Can you work these out from the model? Positions are in its coordinate system, mm. Face numbers are marked on the shaded views. A direction names the side the tool comes from. Coordinates: 2 decimals unless noted, no trailing zeros. Order: outer loops, then holes, each group sorted by start corner. A loop starts at its lowest first (then second) coordinate and runs counter-clockwise, first axis right, second up. Notation, with made-up numbers: (-6.5, -20) -> (14.5, -20) arc R21 ccw to (14.5, -10) -> close; hole circle Ø1 at (88.25, -16). An arc over 180 degrees is marked (long way). Use a Markdown table: item, result. Add a question column.
1. If I drill on line 1 along X through (y, z) = (88.5, 14.75); line 2 along X through (y, z) = (86, 2.75); line 3 along X through (y, z) = (89.5, 4), over which ranges is the centre line in solid material (lowest first)? Write a range as from..to.
2. Suppose I cut it at B-B, the plane z = 17.5. State how many separate pieces and enclosed holes the cut face has, then the cut area to 3 significant figures.
3. For the marked faces 4, 5 and 6, which set-ups out of +Z, -Z, +X, -X, +Y, -Y let a thin tool reach every point of the face, with its end or its side?
4. For pin 1 Ø6 at (y, z) = (92, 15.5) entering from -X; pin 2 Ø3.5 at (x, z) = (12.5, 7) entering from +Y; pin 3 Ø1.5 at (y, z) = (8, 18.5) entering from +X, each with a flat end and sliding along its axis, tell me the tip position at first contact or that it passes through.
5. Suppose I cut it at A-A, the plane y = 115. List the corners of the cut face in (x, z) for me.
6. We'd pull the mould along X, two halves only. Please class the marked faces 1, 2 and 3: pulls with the +X half, pulls with the -X half, needs draft (parallel to the pull), parting line crosses it, or undercut.
```python
from build123d import *

# Parameters (mm, degrees)
BOSS_EXTRUDE1_DEPTH = 25
SKETCH3_W           = 36
SKETCH3_H           = 10
CUT_EXTRUDE1_DEPTH  = 134.88427839
CUT_EXTRUDE2_DEPTH  = 134.88427839
CUT_EXTRUDE3_DEPTH  = 134.88427839
CUT_EXTRUDE4_DEPTH  = 134.88427839
BOSS_EXTRUDE2_DEPTH = 25
BOSS_EXTRUDE3_DEPTH = 25
LPATTERN1_COUNT     = 30
LPATTERN1_PITCH     = 3
CUT_EXTRUDE5_DEPTH  = 138.359842306
CUT_EXTRUDE6_DEPTH  = 138.359842306
CUT_EXTRUDE7_DEPTH  = 138.359842306
CUT_EXTRUDE8_DEPTH  = 138.359842306
CUT_EXTRUDE9_DEPTH  = 138.359842306
FILLET1_R           = 1


with BuildPart() as part:
    # Sketch2 → Boss-Extrude1 (new body)
    with BuildSketch(Plane.XY):
        with BuildLine():
            Line((-15, 0), (15, 0))
            Line((15, 0), (15, 5))
            Line((15, 5), (8, 5))
            Line((8, 5), (8, 10))
            Line((8, 10), (20, 10))
            Line((20, 10), (20, 130))
            ThreePointArc((20, 130), (-9.083269132, 106.055512755), (-20, 70))
            Line((-20, 70), (-20, 10))
            Line((-20, 10), (-8, 10))
            Line((-8, 10), (-8, 5))
            Line((-8, 5), (-15, 5))
            Line((-15, 5), (-15, 0))
        make_face()
    extrude(amount=BOSS_EXTRUDE1_DEPTH)

    # Sketch3 → Cut-Extrude1 (cut, through all)
    with BuildSketch(Plane.XY.offset(25)):
        with Locations((0, 17)):
            Rectangle(SKETCH3_W, SKETCH3_H)
    extrude(amount=-CUT_EXTRUDE1_DEPTH, mode=Mode.SUBTRACT)

    # Sketch4 → Cut-Extrude2 (cut, through all)
    with BuildSketch(Plane.XY.offset(25)):
        Polygon((-18, 24), (18, 24), (18, 34), (-18, 40.347771306), align=None)
    extrude(amount=-CUT_EXTRUDE2_DEPTH, mode=Mode.SUBTRACT)

    # Sketch5 → Cut-Extrude3 (cut, through all)
    with BuildSketch(Plane.XY.offset(25)):
        Polygon((-18, 42.378624529), (18, 36.030853224), (18, 46.030853224), (-18, 59.133781657), align=None)
    extrude(amount=-CUT_EXTRUDE3_DEPTH, mode=Mode.SUBTRACT)

    # Sketch6 → Cut-Extrude4 (cut, through all)
    with BuildSketch(Plane.XY.offset(25)):
        with BuildLine():
            Line((-18, 61.262137202), (18, 48.159208769))
            Line((18, 48.159208769), (18, 58.159208769))
            Line((18, 58.159208769), (-17.409830527, 78.603083956))
            ThreePointArc((-17.409830527, 78.603083956), (-17.852284458, 74.311651469), (-18, 70))
            Line((-18, 70), (-18, 61.262137202))
        make_face()
    extrude(amount=-CUT_EXTRUDE4_DEPTH, mode=Mode.SUBTRACT)

    # Sketch13 → Boss-Extrude2 (add)
    with BuildSketch(Plane.XY.offset(25)):
        with BuildLine():
            Line((28.543587015, 132.015112463), (28.543587015, 130.015112463))
            ThreePointArc((28.543587015, 130.015112463), (22.183163486, 116.610368534), (20, 101.934676234))
            Line((20, 101.934676234), (20, 130))
            ThreePointArc((20, 130), (24.189413282, 131.356828362), (28.543587015, 132.015112463))
        make_face()
    extrude(amount=-BOSS_EXTRUDE2_DEPTH)

    # Sketch15 → Boss-Extrude3 (add)
    with BuildSketch(Plane.XY.offset(25)):
        Polygon((20, 101.934676234), (22.598076211, 100.434676234), (20, 98.934676234), align=None)
    boss_extrude3 = extrude(amount=-BOSS_EXTRUDE3_DEPTH)

    # LPattern1: Boss-Extrude3 ×30
    with Locations(*[(0, -i * LPATTERN1_PITCH, 0) for i in range(1, LPATTERN1_COUNT)]):
        add(boss_extrude3)

    # Sketch17 → Cut-Extrude5 (cut, through all)
    with BuildSketch(Plane.XY.offset(25)):
        with BuildLine():
            Line((-17.080813578, 80.722527008), (18, 60.468609845))
            Line((18, 60.468609845), (18, 70.468609845))
            Line((18, 70.468609845), (-12.396357526, 95.974182235))
            ThreePointArc((-12.396357526, 95.974182235), (-15.223349712, 88.497247077), (-17.080813578, 80.722527008))
        make_face()
    extrude(amount=-CUT_EXTRUDE5_DEPTH, mode=Mode.SUBTRACT)

    # Sketch18 → Cut-Extrude6 (cut, through all)
    with BuildSketch(Plane.XY.offset(25)):
        with BuildLine():
            Line((-11.513032555, 97.843799156), (18, 73.079424424))
            Line((18, 73.079424424), (18, 83.079424424))
            Line((18, 83.079424424), (-4.123287406, 109.44493167))
            ThreePointArc((-4.123287406, 109.44493167), (-8.135718614, 103.846645438), (-11.513032555, 97.843799156))
        make_face()
    extrude(amount=-CUT_EXTRUDE6_DEPTH, mode=Mode.SUBTRACT)

    # Sketch19 → Cut-Extrude7 (cut, through all)
    with BuildSketch(Plane.XY.offset(25)):
        with BuildLine():
            Line((-2.825102167, 111.009262402), (18, 86.190872078))
            Line((18, 86.190872078), (18, 96.190872078))
            Line((18, 96.190872078), (5.013768012, 118.68368568))
            ThreePointArc((5.013768012, 118.68368568), (0.926972027, 115.017421131), (-2.825102167, 111.009262402))
        make_face()
    extrude(amount=-CUT_EXTRUDE7_DEPTH, mode=Mode.SUBTRACT)

    # Sketch21 → Cut-Extrude8 (cut, through all)
    with BuildSketch(Plane.XY.offset(25)):
        with BuildLine():
            Line((6.596754137, 119.941873284), (18, 100.190872078))
            Line((18, 100.190872078), (18, 110.190872078))
            Line((18, 110.190872078), (12.898276405, 124.207742456))
            ThreePointArc((12.898276405, 124.207742456), (9.683048128, 122.170038436), (6.596754137, 119.941873284))
        make_face()
    extrude(amount=-CUT_EXTRUDE8_DEPTH, mode=Mode.SUBTRACT)

    # Sketch22 → Cut-Extrude9 (cut, through all)
    with BuildSketch(Plane.XY.offset(25)):
        with BuildLine():
            Line((14.660598632, 125.213410732), (18, 116.038480878))
            Line((18, 116.038480878), (18, 126.920997883))
            ThreePointArc((18, 126.920997883), (16.317589, 126.092060929), (14.660598632, 125.213410732))
        make_face()
    extrude(amount=-CUT_EXTRUDE9_DEPTH, mode=Mode.SUBTRACT)

    # Fillet1
    fillet1_edges = [part.edges().sort_by_distance(p)[0] for p in [
        (18, 70.468609845, 12.5),
        (18, 60.468609845, 12.5),
        (-17.080813578, 80.722527008, 12.5),
        (-12.396357526, 95.974182235, 12.5),
        (-11.513032555, 97.843799156, 12.5),
        (-4.123287406, 109.44493167, 12.5),
        (18, 83.079424424, 12.5),
        (18, 73.079424424, 12.5),
        (18, 96.190872078, 12.5),
        (18, 86.190872078, 12.5),
        (-2.825102167, 111.009262402, 12.5),
        (5.013768012, 118.68368568, 12.5),
        (6.596754137, 119.941873284, 12.5),
        (12.898276405, 124.207742456, 12.5),
        (18, 110.190872078, 12.5),
        (18, 100.190872078, 12.5),
        (14.660598632, 125.213410732, 12.5),
        (18, 126.920997883, 12.5),
        (18, 116.038480878, 12.5),
        (-18, 12, 12.5),
        (-18, 22, 12.5),
        (18, 22, 12.5),
        (18, 12, 12.5),
        (-18, 24, 12.5),
        (-18, 40.347771306, 12.5),
        (18, 34, 12.5),
        (18, 24, 12.5),
        (-18, 42.378624529, 12.5),
        (-18, 59.133781657, 12.5),
        (18, 46.030853224, 12.5),
        (18, 36.030853224, 12.5),
        (-18, 61.262137202, 12.5),
        (-17.409830527, 78.603083956, 12.5),
        (18, 58.159208769, 12.5),
        (18, 48.159208769, 12.5),
    ]]
    fillet(fillet1_edges, radius=FILLET1_R)


solid = part.part
```
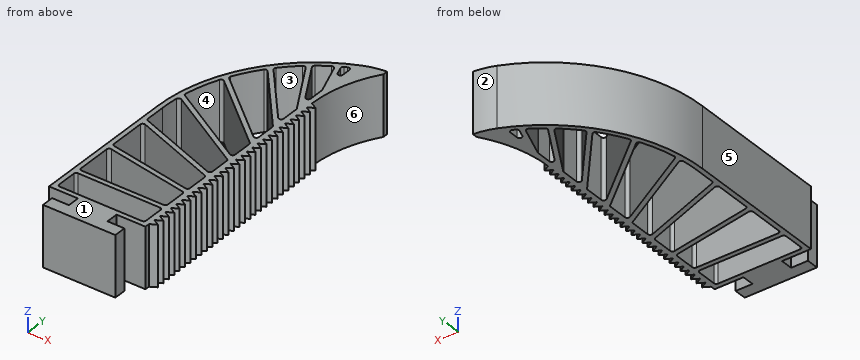
Worked out:
| question | item | result |
|---|---|---|
| 1 | line 1 | x = -17.31..-15.22, -3.49..-0.38, 13.45..16.06, 17.9..22.48 |
| 1 | line 2 | x = -18..-15.93, -0.51..2.6, 15.55..21.62 |
| 1 | line 3 | x = -17.01..-14.91, -4.68..-1.57, 12.61..15.22, 18..20.75 |
| 2 | separate pieces | 1 |
| 2 | enclosed holes | 9 |
| 2 | area | 1,550 mm² |
| 3 | face 4 | +Z, -Z |
| 3 | face 5 | +Z, -Z, -X, +Y, -Y |
| 3 | face 6 | +Z, -Z, +X |
| 4 | pin 1 | stops at x = -17.16 |
| 4 | pin 2 | stops at y = 127.27 |
| 4 | pin 3 | stops at x = 8 |
| 5 | outline | (-1.9, 0) -> (0.91, 0) -> (0.91, 25) -> (-1.9, 25) -> close; (7.14, 0) -> (9.45, 0) -> (9.45, 25) -> (7.14, 25) -> close; (16.25, 0) -> (21.72, 0) -> (21.72, 25) -> (16.25, 25) -> close |
| 6 | face 1 | needs draft |
| 6 | face 2 | pulls with the -X half |
| 6 | face 3 | undercut |
